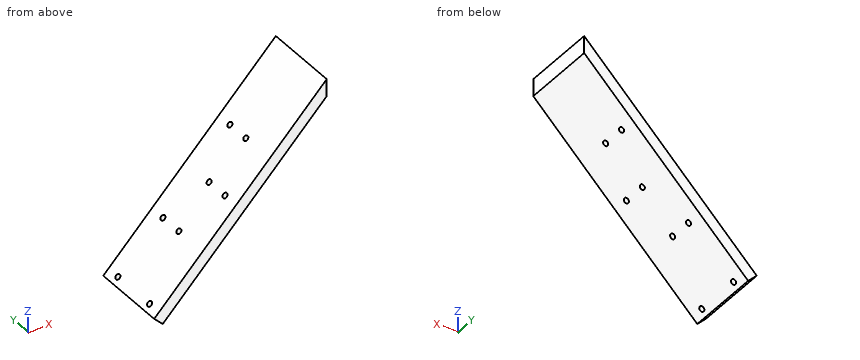
from build123d import *

# Parameters (mm, degrees)
BOSS_EXTRUDE1_DEPTH = 32
FILLET1_R           = 10
SKETCH4_W           = 170.11041037
SKETCH4_H           = 258.008077424
CUT_EXTRUDE2_DEPTH  = 33
SKETCH5_R           = 1.1
CUT_EXTRUDE3_DEPTH  = 57.514129524
SKETCH6_R           = 1.1
CUT_EXTRUDE4_DEPTH  = 57.514129524


with BuildPart() as part:
    # Sketch1 → Boss-Extrude1 (new body)
    with BuildSketch(Plane(origin=(0, 0, 0), x_dir=(1, 0, 0), z_dir=(0, 1, 0))):
        Polygon((0, 0), (0, 30), (83, 115), (83, 107.843231513), (5, 27.963713441), (5, -27.963713441), (83, -107.843231513), (83, -115), (0, -30), align=None)
    extrude(amount=BOSS_EXTRUDE1_DEPTH)

    # Fillet1
    fillet1_edges = [part.edges().sort_by_distance(p)[0] for p in [
        (0, 16, 30),
        (0, 16, -30),
    ]]
    fillet(fillet1_edges, radius=FILLET1_R)

    # Sketch4 → Cut-Extrude2 (cut, through all)
    with BuildSketch(Plane(origin=(0, 32, 0), x_dir=(1, 0, 0), z_dir=(0, 1, 0))):
        with Locations((35.635219957, -4.046970822)):
            Rectangle(SKETCH4_W, SKETCH4_H)
        Polygon((14.577370106, -37.771863549), (86.577370106, -111.506803308), (83, -115), (11, -41.265060241), align=None, mode=Mode.SUBTRACT)
    extrude(amount=-CUT_EXTRUDE2_DEPTH, mode=Mode.SUBTRACT)

    # Sketch5 → Cut-Extrude3 (cut, through all)
    with BuildSketch(Plane(origin=(-11.418378796, 0, 11.14971106), x_dir=(-0.698639338, 0, -0.715474021), z_dir=(0.715474021, 0, -0.698639338))):
        with Locations((-40.209111306, 26)):
            Circle(SKETCH5_R)
        with Locations((-40.209111306, 6)):
            Circle(SKETCH5_R)
    extrude(amount=-CUT_EXTRUDE3_DEPTH, mode=Mode.SUBTRACT)

    # Sketch6 → Cut-Extrude4 (cut, through all)
    with BuildSketch(Plane(origin=(-11.418378796, 0, 11.14971106), x_dir=(-0.698639338, 0, -0.715474021), z_dir=(0.715474021, 0, -0.698639338))):
        with Locations((-66.177603446, 25)):
            Circle(SKETCH6_R)
        with Locations((-66.177603446, 15)):
            Circle(SKETCH6_R)
        with Locations((-106.177603446, 15)):
            Circle(SKETCH6_R)
        with Locations((-106.177603446, 25)):
            Circle(SKETCH6_R)
        with Locations((-86.177603446, 17)):
            Circle(SKETCH6_R)
        with Locations((-86.177603446, 7)):
            Circle(SKETCH6_R)
    extrude(amount=-CUT_EXTRUDE4_DEPTH, mode=Mode.SUBTRACT)


solid = part.part
Design review of the part built by this model. Coordinates are the model's own, in mm. Coordinates: 2 decimals unless noted, no trailing zeros. Loops run counter-clockwise (first coordinate to the right, second up) from the corner with the lowest first, then second, coordinate; pieces in that order, holes last.
Item 1: Clearance check with flat-ended pins moving along their axes: pin 1 (1 mm diameter, centred on x = 30.5, y = 21.5, fed in from -Z); pin 2 (1.5 mm diameter, centred on x = 70.5, z = 106, fed in from -Y); pin 3 (12 mm diameter, centred on y = 3.5, z = 93.5, fed in from -X); pin 4 (5 mm diameter, centred on x = 24, y = 24.5, fed in from -Z). State where each tip first meets the part, or that it passes through.
Completed:
pin 1: stops at z = 53.57
pin 2: passes through
pin 3: stops at x = 56.15
pin 4: stops at z = 44.86
Item 2: Wall thickness on L1, parallel to X at y = 1.5, z = 83; L2, parallel to X at y = 4.5, z = 48.5; L3, parallel to Z at x = 79, y = 29.5: over which ranges is each line inside the solid? List them lowest first.
Completed:
L1: x = 51.75 to 58.74
L2: x = 18.06 to 25.05
L3: z = 103.75 to 110.9
Item 3: Add section B-B (x = 43). Write out the cut boundary in (y, z).
Completed:
outline: (0, 66.88) - (32, 66.88) - (32, 74.04) - (0, 74.04) - close
Item 4: Add section C-C (x = 60). Give the number of separate pieces and of enclosed holes in the cut face, and give its area (3 significant figures).
Completed:
separate pieces: 1
enclosed holes: 2
area: 218 mm2
Item 5: Add section A-A (y = 22). Write out the cut boundary in (x, z).
Completed:
outline: (11, 41.27) - (14.58, 37.77) - (83, 107.84) - (83, 115) - close
